Here's the drawing with two shaded views (mm, measured from the low corner). I have some questions. Coordinates: 2 decimals unless noted, no trailing zeros. Write each loop counter-clockwise with the first axis right and the second up, starting at its lowest first coordinate (ties: lowest second). Pieces come first, ordered by that corner, then holes. Notation, with made-up numbers: (32.25, 80) -> (54.25, 80) arc R18 cw to (54.25, 94) -> close; hole circle Ø2 at (-38.75, 63.5). An arc over 180 degrees is marked (long way). Use one line per item in the form item = value.
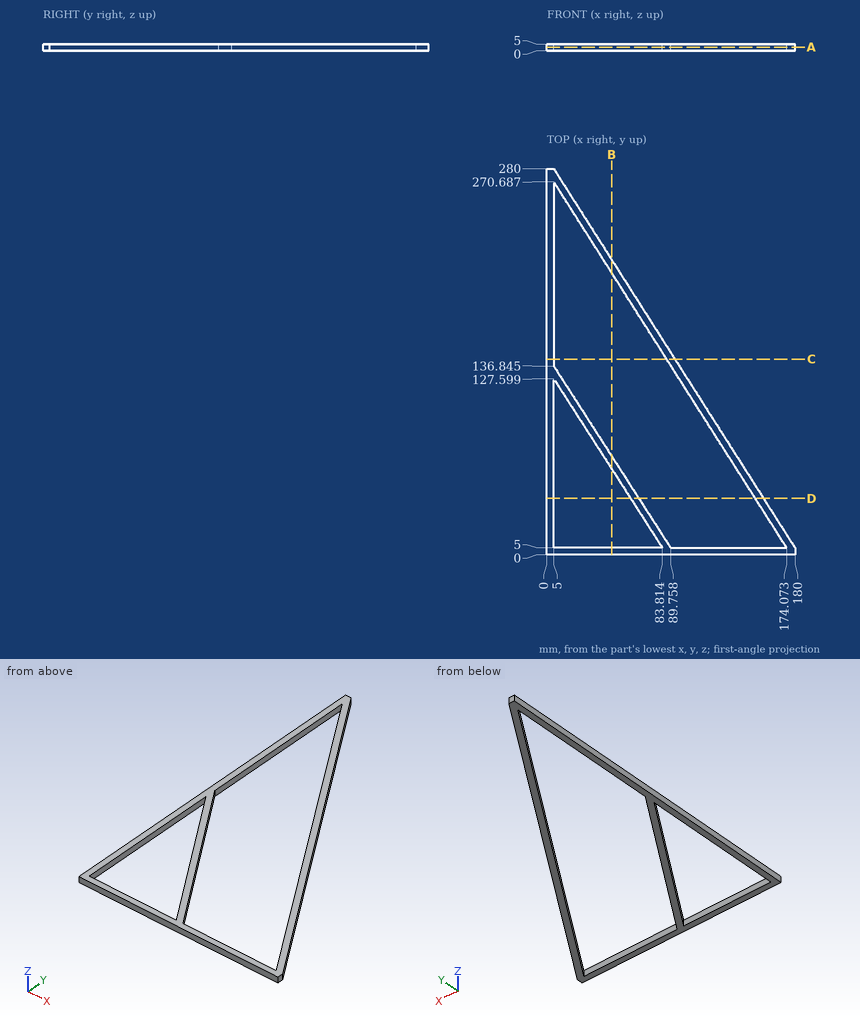
Q1. Suppose I cut it at D-D (y = 41). Write out the boundary of the cut face in (x, z) (1 decimal).
Return value:
outline = (0, 0) -> (5, 0) -> (5, 5) -> (0, 5) -> close; (60.7, 0) -> (66.6, 0) -> (66.6, 5) -> (60.7, 5) -> close; (151.2, 0) -> (157.1, 0) -> (157.1, 5) -> (151.2, 5) -> close
Q2. Will these pins go through, and if not, where does the flat tip stop? pin 1 (2.5 mm diameter, centred on y = 217, z = 2, fed in from +X); pin 2 (1.5 mm diameter, centred on x = 37, z = 2.5, fed in from +Y) (1 decimal); pin 3 (2.5 mm diameter, centred on y = 89.5, z = 3, fed in from +X).
Return value:
pin_1 = 45.89
pin_2 = 230.9
pin_3 = 127.02
Q3. If I drill on line 1 (X direction, y = 73, z = 0.2) (1 decimal); line 2 (Y direction, x = 57.5, z = 4.2) (1 decimal); line 3 (Y direction, x = 9, z = 2.1) (1 decimal), over which ranges is the centre line in solid material (lowest first)? Write a range as from..to.
Return value:
line_1 = 0..5, 40.1..46, 130.8..136.7
line_2 = 0..5, 45.9..55.2, 188.2..197.5
line_3 = 0..5, 121.4..130.6, 264.4..273.7
Q4. Suppose I cut it at C-C (y = 142). Write out the boundary of the cut face in (x, z).
Return value:
outline = (0, 0) -> (5, 0) -> (5, 5) -> (0, 5) -> close; (86.89, 0) -> (92.82, 0) -> (92.82, 5) -> (86.89, 5) -> close
Q5. Suppose I cut it at A-A (z = 2.65). Write out the boundary of the cut face in (x, y) (1 decimal).
Return value:
outline = (0, 0) -> (180, 0) -> (180, 5) -> (5, 280) -> (0, 280) -> close; hole (5, 5) -> (83.8, 5) -> (5, 127.6) -> close; hole (5, 136.8) -> (89.8, 5) -> (174.1, 5) -> (5, 270.7) -> close
Q6. Suppose I cut it at B-B (x = 47). Write out the boundary of the cut face in (y, z) (1 decimal).
Return value:
outline = (0, 0) -> (5, 0) -> (5, 5) -> (0, 5) -> close; (62.3, 0) -> (71.5, 0) -> (71.5, 5) -> (62.3, 5) -> close; (204.7, 0) -> (214, 0) -> (214, 5) -> (204.7, 5) -> close
